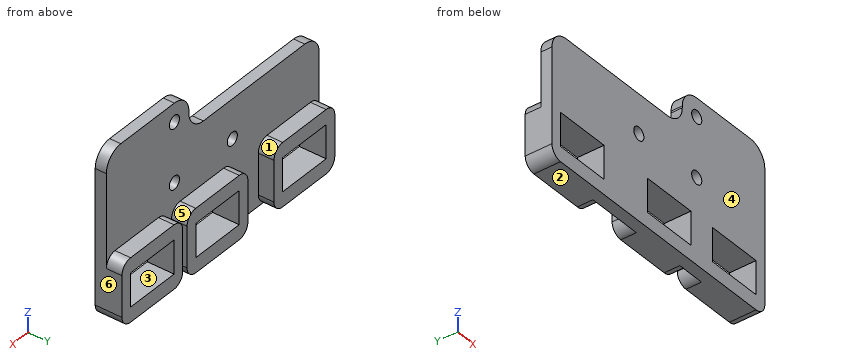
from build123d import *

# Parameters (mm, degrees)
SKETCH_1_W          = 21
SKETCH_1_H          = 17
SKETCH_1_W_2        = 15
SKETCH_1_H_2        = 9
EXTRUDE_1_DEPTH     = 4.2
EXTRUDE_1_2_DEPTH   = 4.2
EXTRUDE_1_3_DEPTH   = 4.2
SKETCH_2_W          = 73.5
SKETCH_2_H          = 44
SKETCH_2_R          = 1.75
SKETCH_2_W_2        = 15
SKETCH_2_H_2        = 9
EXTRUDE_2_DEPTH     = 3
FILLET_1_R          = 3
SKETCH_3_W          = 45
SKETCH_3_H          = 10.5
CUT_EXTRUDE_1_DEPTH = 56.196376693
FILLET_2_R          = 5


with BuildPart() as part:
    # Sketch 1 → Extrude 1 (new body)
    with BuildSketch(Plane(origin=(0, 0, 0), x_dir=(1, 0, 0), z_dir=(0, 1, 0))):
        with Locations((13, 14.5)):
            Rectangle(SKETCH_1_W, SKETCH_1_H)
        with Locations((13, 14.5)):
            Rectangle(SKETCH_1_W_2, SKETCH_1_H_2, mode=Mode.SUBTRACT)
    extrude(amount=EXTRUDE_1_DEPTH)



with BuildPart() as body_2:
    # Sketch 1 → Extrude 1 2 (new body)
    with BuildSketch(Plane(origin=(0, 0, 0), x_dir=(1, 0, 0), z_dir=(0, 1, 0))):
        with Locations((-9.5, 14.5)):
            Rectangle(SKETCH_1_W, SKETCH_1_H)
        with Locations((-9.5, 14.5)):
            Rectangle(SKETCH_1_W_2, SKETCH_1_H_2, mode=Mode.SUBTRACT)
    extrude(amount=EXTRUDE_1_2_DEPTH)


with BuildPart() as body_3:
    # Sketch 1 → Extrude 1 3 (new body)
    with BuildSketch(Plane(origin=(0, 0, 0), x_dir=(1, 0, 0), z_dir=(0, 1, 0))):
        with Locations((-39.5, 14.5)):
            Rectangle(SKETCH_1_W, SKETCH_1_H)
        with Locations((-39.5, 14.5)):
            Rectangle(SKETCH_1_W_2, SKETCH_1_H_2, mode=Mode.SUBTRACT)
    extrude(amount=EXTRUDE_1_3_DEPTH)


with BuildPart() as part_1:
    add(part.part)

    add(body_2.part)  # Extrude 2 merges body 2

    add(body_3.part)  # Extrude 2 merges body 3
    # Sketch 2 → Extrude 2 (add)
    with BuildSketch(Plane.XZ):
        with Locations((-13.25, -1)):
            Rectangle(SKETCH_2_W, SKETCH_2_H)
        with Locations(Location((0, 0, 0), (0, 0, 270))):
            Circle(SKETCH_2_R, mode=Mode.SUBTRACT)
        with Locations(Location((0, 16, 0), (0, 0, 270))):
            Circle(SKETCH_2_R, mode=Mode.SUBTRACT)
        with Locations(Location((-20, 0, 0), (0, 0, 270))):
            Circle(SKETCH_2_R, mode=Mode.SUBTRACT)
        with Locations((-39.5, -14.5)):
            Rectangle(SKETCH_2_W_2, SKETCH_2_H_2, mode=Mode.SUBTRACT)
        with Locations((-9.5, -14.5)):
            Rectangle(SKETCH_2_W_2, SKETCH_2_H_2, mode=Mode.SUBTRACT)
        with Locations((13, -14.5)):
            Rectangle(SKETCH_2_W_2, SKETCH_2_H_2, mode=Mode.SUBTRACT)
    extrude(amount=EXTRUDE_2_DEPTH)

    # Fillet 1
    fillet_1_edges = [part_1.edges().sort_by_distance(p)[0] for p in [
        (1, 2.1, -23),
        (-20, 2.1, -23),
        (-20, 2.1, -6),
        (1, 2.1, -6),
        (-29, 2.1, -23),
        (-50, 2.1, -6),
        (-29, 2.1, -6),
        (-50, 0.6, -23),
        (23.5, 2.1, -6),
        (2.5, 2.1, -6),
        (2.5, 2.1, -23),
        (23.5, 0.6, -23),
    ]]
    fillet(fillet_1_edges, radius=FILLET_1_R)

    # Sketch 3 → Cut-Extrude 1 (cut, through all)
    with BuildSketch(Plane(origin=(0, 0, 0), x_dir=(1, 0, 0), z_dir=(0, 1, 0))):
        with Locations((-27.5, -15.75)):
            Rectangle(SKETCH_3_W, SKETCH_3_H)
    extrude(amount=-CUT_EXTRUDE_1_DEPTH, mode=Mode.SUBTRACT)

    # Fillet 2
    fillet_2_edges = [part_1.edges().sort_by_distance(p)[0] for p in [
        (-50, -1.5, 10.5),
        (-5, -1.5, 10.5),
        (-5, -1.5, 21),
        (23.5, -1.5, 21),
    ]]
    fillet(fillet_2_edges, radius=FILLET_2_R)


solid = part_1.part
Design review of the part built by this model. Coordinates are the model's own, in mm. Face numbers are marked on the shaded views. A direction names the side the tool comes from. Round coordinates to 2 decimals unless told otherwise and drop trailing zeros. Loops run counter-clockwise (first coordinate to the right, second up) from the corner with the lowest first, then second, coordinate; pieces in that order, holes last. Notation, with made-up numbers: M 28.5,-38.75 L 46.5,-38.75 A19 cw 46.5,-29.75 Z; hole C -8,20 d6. An arc over 180 degrees is marked long. Answer as a JSON object with one key per item and string values.
Item 1: The part is to be moulded in two halves that separate along X. For the marked faces 4, 5 and 6, say which applies: pulls with the +X half, pulls with the -X half, needs draft (parallel to the pull), parting line crosses it, or undercut.
Answer sheet:
{"face 4": "needs draft", "face 5": "undercut", "face 6": "pulls with the +X half"}
Item 2: Wall thickness on L1, parallel to X at y = -1.3, z = 0; L2, parallel to X at y = 1, z = -20; L3, parallel to X at y = -1.1, z = 16: over which ranges is each line inside the solid? List them lowest first. Write a range as from..to.
Answer sheet:
{"L1": "x = -50..-21.75, -18.25..-1.75, 1.75..23.5", "L2": "x = -50..-29, -20..1, 2.5..23.5", "L3": "x = -5..-1.75, 1.75..23.5"}
Item 3: We need section D-D on z = 0. Give the boundary of the cut face in (x, y), and give its area (4 significant figures).
Answer sheet:
{"outline": "M -50,-3 L -21.75,-3 L -21.75,0 L -50,0 Z; M -18.25,-3 L -1.75,-3 L -1.75,0 L -18.25,0 Z; M 1.75,-3 L 23.5,-3 L 23.5,0 L 1.75,0 Z", "area": "199.5 mm^2"}
Item 4: Clearance check with flat-ended pins moving along their axes: P1, Ø1.3, axis at x = 16, y = 2.5, coming from the +Z side; P2, Ø3, axis at x = 0, z = 16, coming from the -Y side; P3, Ø2.5, axis at x = -19.5, y = -1.5, coming from the +Z side; P4, Ø1.5, axis at x = -21, z = -5.5, coming from the +Y side. State where each tip first meets the part, or that it passes through.
Answer sheet:
{"P1": "stops at z = -6", "P2": "passes through", "P3": "stops at z = 10.5", "P4": "stops at y = 0"}
Item 5: We need section A-A on x = 11.5. Give the boundary of the cut face in (y, z).
Answer sheet:
{"outline": "M -3,-23 L 4.2,-23 L 4.2,-19 L -3,-19 Z; M -3,-10 L 4.2,-10 L 4.2,-6 L 0,-6 L 0,21 L -3,21 Z"}
Item 6: Machinability: for the marked faces 1, 2 and 3, which of the approach directions +Z, -Z, +X, -X, +Y, -Y give a long, thin tool a straight path to every point of the face, cutting with its end or side? Answer none if there is none.
Answer sheet:
{"face 1": "+Z, +Y", "face 2": "-Z, +X, -X, +Y, -Y", "face 3": "+Y, -Y"}
Item 7: We need section B-B on z = -18. Give the boundary of the cut face in (x, y).
Answer sheet:
{"outline": "M -50,-3 L -47,-3 L -47,4.2 L -50,4.2 Z; M -32,-3 L -17,-3 L -17,4.2 L -20,4.2 L -20,0 L -29,0 L -29,4.2 L -32,4.2 Z; M -2,-3 L 5.5,-3 L 5.5,4.2 L 2.5,4.2 L 2.5,0 L 1,0 L 1,4.2 L -2,4.2 Z; M 20.5,-3 L 23.5,-3 L 23.5,4.2 L 20.5,4.2 Z"}
Item 8: We need section C-C on y = 3.5. State how many separate pieces and enclosed holes the cut face has, and give its area (3 significant figures).
Answer sheet:
{"separate pieces": "3", "enclosed holes": "3", "area": "643 mm^2"}
